from build123d import *

# Parameters (mm, degrees)
CSK_FOR_M2_5_FLAT_HEAD_MACHINE_SCREW1_D           = 2.9
CSK_FOR_M2_5_FLAT_HEAD_MACHINE_SCREW1_CSINK_D     = 5.5
CSK_FOR_M2_5_FLAT_HEAD_MACHINE_SCREW1_CSINK_ANGLE = 90
F_5_0_2055_DIAMETER_HOLE1_AT_2_COUNT              = 2
F_5_0_2055_DIAMETER_HOLE1_AT_2_PITCH              = 12.7
CHAMFER1_SIZE                                     = 4.7625
CHAMFER1_SIZE2                                    = 0.669325725
CHAMFER1_PART_2_SIZE                              = 4.7625
CHAMFER1_PART_2_SIZE2                             = 0.669325725
CIRPATTERN3_COUNT                                 = 4
CHAMFER1_OF_CIRPATTERN3_SIZE2                     = 4.7625
CHAMFER1_OF_CIRPATTERN3_SIZE                      = 0.669325725
CHAMFER1_PART_2_OF_CIRPATTERN3_SIZE2              = 4.7625
CHAMFER1_PART_2_OF_CIRPATTERN3_SIZE               = 0.669325725
FILLET10_R                                        = 6.35


with BuildPart() as part:
    # Sketch32 → Revolve8 (revolve)
    with BuildSketch(Plane(origin=(0, 0, 0), x_dir=(0, 0, -1), z_dir=(1, 0, 0))):
        Polygon((-38.1, 0), (-38.1, 19.05), (-6.35, 38.1), (0, 38.1), (0, 0), align=None)
    revolve(axis=Axis((0, 0, 0), (0, 0, 1)))

    # Sketch33 → Cut-Revolve1 (revolve, cut)
    with BuildSketch(Plane(origin=(0, 0, 0), x_dir=(0, 0, -1), z_dir=(1, 0, 0))):
        Polygon((-31.75, 14.2875), (-31.75, 4), (-38.1, 4), (-38.1, 0), (0, 0), (0, 14.2875), align=None)
    revolve(axis=Axis((0, 0, 0), (0, 0, 1)), mode=Mode.SUBTRACT)

    # CSK for M2.5 Flat Head Machine Screw1 (through all)
    with Locations(Plane.XY.offset(38.1)):
        with Locations((0, 7.5), (0, -7.5)):
            CounterSinkHole(CSK_FOR_M2_5_FLAT_HEAD_MACHINE_SCREW1_D / 2, CSK_FOR_M2_5_FLAT_HEAD_MACHINE_SCREW1_CSINK_D / 2, counter_sink_angle=CSK_FOR_M2_5_FLAT_HEAD_MACHINE_SCREW1_CSINK_ANGLE)

    # Sketch40 → 5 _0.2055_ Diameter Hole1 (revolve, cut)
    with BuildSketch(Plane(origin=(-6.35, 28.511429287, 0), x_dir=(0, 1, 0), z_dir=(1, 0, 0))):
        Polygon((0, 0), (0, 11.093156087), (2.60985, 9.525), (2.60985, 0), align=None)
    f_5_0_2055_diameter_hole1 = revolve(axis=Axis((-6.35, 28.511429287, -6.35), (0, 0, 1)), mode=Mode.SUBTRACT)

    # 5 _0.2055_ Diameter Hole1 at 2: 5 _0.2055_ Diameter Hole1 ×2
    with Locations(*[(i * F_5_0_2055_DIAMETER_HOLE1_AT_2_PITCH, 0, 0) for i in range(1, F_5_0_2055_DIAMETER_HOLE1_AT_2_COUNT)]):
        add(f_5_0_2055_diameter_hole1, mode=Mode.SUBTRACT)

    # Chamfer1
    chamfer1_edges = [part.edges().sort_by_distance(p)[0] for p in [
        (-6.35, 25.901579287, 0),
    ]]
    chamfer1_side = [part.faces().sort_by_distance(p)[0] for p in [
        (-6.35, 25.901579287, 4.7625),
    ]]
    chamfer(chamfer1_edges, length=CHAMFER1_SIZE, length2=CHAMFER1_SIZE2, reference=chamfer1_side[0])

    # Chamfer1 part 2
    chamfer1_part_2_edges = [part.edges().sort_by_distance(p)[0] for p in [
        (6.35, 25.901579287, 0),
    ]]
    chamfer1_part_2_side = [part.faces().sort_by_distance(p)[0] for p in [
        (6.35, 25.901579287, 4.7625),
    ]]
    chamfer(chamfer1_part_2_edges, length=CHAMFER1_PART_2_SIZE, length2=CHAMFER1_PART_2_SIZE2, reference=chamfer1_part_2_side[0])

    # CirPattern3: 5 _0.2055_ Diameter Hole1 ×4 about axis
    cirpattern3_axis = Axis((0, 0, 0), (0, 0, 1))
    for i in range(1, CIRPATTERN3_COUNT):
        add(f_5_0_2055_diameter_hole1.rotate(cirpattern3_axis, i * 360 / CIRPATTERN3_COUNT), mode=Mode.SUBTRACT)

    # CirPattern3 copy 1 sketch → CirPattern3 copy 1 (revolve, cut)
    with BuildSketch(Plane(origin=(-28.511429287, 6.35, 0), x_dir=(-1, 0, 0), z_dir=(0, 1, 0))):
        Polygon((0, 0), (0, 11.093156087), (2.60985, 9.525), (2.60985, 0), align=None)
    revolve(axis=Axis((-28.511429287, 6.35, -6.35), (0, 0, 1)), mode=Mode.SUBTRACT)

    # CirPattern3 copy 2 sketch → CirPattern3 copy 2 (revolve, cut)
    with BuildSketch(Plane(origin=(-6.35, -28.511429287, 0), x_dir=(0, -1, 0), z_dir=(-1, 0, 0))):
        Polygon((0, 0), (0, 11.093156087), (2.60985, 9.525), (2.60985, 0), align=None)
    revolve(axis=Axis((-6.35, -28.511429287, -6.35), (0, 0, 1)), mode=Mode.SUBTRACT)

    # CirPattern3 copy 3 sketch → CirPattern3 copy 3 (revolve, cut)
    with BuildSketch(Plane(origin=(28.511429287, -6.35, 0), x_dir=(1, 0, 0), z_dir=(0, -1, 0))):
        Polygon((0, 0), (0, 11.093156087), (2.60985, 9.525), (2.60985, 0), align=None)
    revolve(axis=Axis((28.511429287, -6.35, -6.35), (0, 0, 1)), mode=Mode.SUBTRACT)

    # Chamfer1 of CirPattern3
    chamfer1_of_cirpattern3_edges = [part.edges().sort_by_distance(p)[0] for p in [
        (-25.901579287, -6.35, 0),
        (6.35, -25.901579287, 0),
        (25.901579287, 6.35, 0),
    ]]
    chamfer(chamfer1_of_cirpattern3_edges, length=CHAMFER1_OF_CIRPATTERN3_SIZE, length2=CHAMFER1_OF_CIRPATTERN3_SIZE2)

    # Chamfer1 part 2 of CirPattern3
    chamfer1_part_2_of_cirpattern3_edges = [part.edges().sort_by_distance(p)[0] for p in [
        (-25.901579287, 6.35, 0),
        (-6.35, -25.901579287, 0),
        (25.901579287, -6.35, 0),
    ]]
    chamfer(chamfer1_part_2_of_cirpattern3_edges, length=CHAMFER1_PART_2_OF_CIRPATTERN3_SIZE, length2=CHAMFER1_PART_2_OF_CIRPATTERN3_SIZE2)

    # Fillet10
    fillet10_edges = [part.edges().sort_by_distance(p)[0] for p in [
        (0, -38.1, 6.35),
        (0, -19.05, 38.1),
    ]]
    fillet(fillet10_edges, radius=FILLET10_R)


solid = part.part
Work out the finished part from the listing and answer in its coordinate system (mm). A direction names the side the tool comes from. Give positions to 0.01 mm unless a question says otherwise; leave off trailing zeros. Order: outer loops, then holes, each group sorted by start corner. A loop starts at its lowest first (then second) coordinate and runs counter-clockwise, first axis right, second up. Notation, with made-up numbers: (85.5, 75) -> (108.5, 75) arc R9 cw to (108.5, 84) -> close; hole circle Ø2 at (34.5, 36.25). An arc over 180 degrees is marked (long way). Answer as a JSON object with one key per item and string values. Group by question number.
1. The mould has two halves that part along X. Classify faces 1 (the cylindrical face through (23.183, -30.235, 2.263)), 2 (the conical face through (-3.93, -30.05, 2.94)): released by +X, released by -X, zero draft, split by the parting line, or undercut.
2. Flat-ended cylindrical pins translate along their axes: pin 1 Ø7 at (x, y) = (6.35, -28.51) entering from -Z; pin 2 Ø2 at (x, z) = (4, 8) entering from -Y; pin 3 Ø7 at (x, y) = (28.51, -6.35) entering from +Z; pin 4 Ø1.5 at (x, z) = (-10, 9) entering from -Y. Find the tip coordinate at first contact, or state that the pin passes through.
3. Section B-B on z = 34 is taken. Determine the outline of the cut face in (x, y).
4. Section A-A on z = 20 is taken. Determine the outline of the cut face in (x, y) (1 decimal).
5. A tool of negligible diameter and unlimited length cuts with its end or side. For faces 3 (the cylindrical face through (-8.114, 26.588, 7.11)), 4 (the cylindrical face through (3.905, -0.867, 34.969)), from which of +Z, -Z, +X, -X, +Y, -Y can it reach the whole face along a straight path? Write none if from no direction.
6. Section C-C on z = 27 is taken. Determine the outline of the cut face in (x, y) (1 decimal), plus the area to 3 significant figures.
7. Consider line 1 along Y through (x, z) = (8, 8); line 2 along X through (y, z) = (7.5, 33.4); line 3 along Y through (x, z) = (0, 32.8). Determine where each line is inside the solid, lowest interval first. Write a range as [from, to].
Result sheet:
{
 "1": {"face 1": "split by the parting line", "face 2": "undercut"},
 "2": {"pin 1": "stops at z = 0", "pin 2": "stops at y = -37.42", "pin 3": "stops at z = 27", "pin 4": "stops at y = -35.63"},
 "3": {"outline": "circle Ø43.02 at (0, 0); hole circle Ø8 at (0, 0); hole circle Ø2.9 at (0, -7.5); hole circle Ø2.9 at (0, 7.5)"},
 "4": {"outline": "circle Ø59.8 at (0, 0); hole circle Ø28.6 at (0, 0)"},
 "5": {"face 3": "-Z", "face 4": "+Z, -Z"},
 "6": {"outline": "circle Ø51.4 at (0, 0); hole circle Ø28.6 at (0, 0)", "area": "1,440 mm^2"},
 "7": {"line 1": "y = [-36.24, -30.53], [-26.49, -11.84], [11.84, 26.49], [30.53, 36.24]", "line 2": "x = [-20.54, -1.45], [1.45, 20.54]", "line 3": "y = [-22.23, -8.95], [-6.05, -4], [4, 6.05], [8.95, 22.23]"}
}
